Geometry: final body of the model. Coordinates: model frame, mm. Give positions to 0.01 mm unless a question says otherwise; leave off trailing zeros. Loops run counter-clockwise (first coordinate to the right, second up) from the corner with the lowest first, then second, coordinate; pieces in that order, holes last.
1. First-contact query: P1, Ø10, axis at y = 17, z = 9.5, coming from the -X side; P2, Ø8, axis at x = 371, z = 9, coming from the +Y side; P3, Ø4, axis at y = -11.5, z = 5.5, coming from the -X side. Flat tips, straight axial feed; report the tip coordinate or a pass-through.
2. Section A-A, the plane z = 19. Output: boundary loops of the cut face in (x, y).
3. Section B-B, the plane x = 319. Output: boundary loops of the cut face in (y, z), then the cut area to 3 significant figures.
4. Material intervals for line 1 along Y through (x, z) = (102.5, 24.5); line 2 along X through (y, z) = (-8, 21.25); line 3 along X through (y, z) = (1.5, 11.5), sorted ascending.
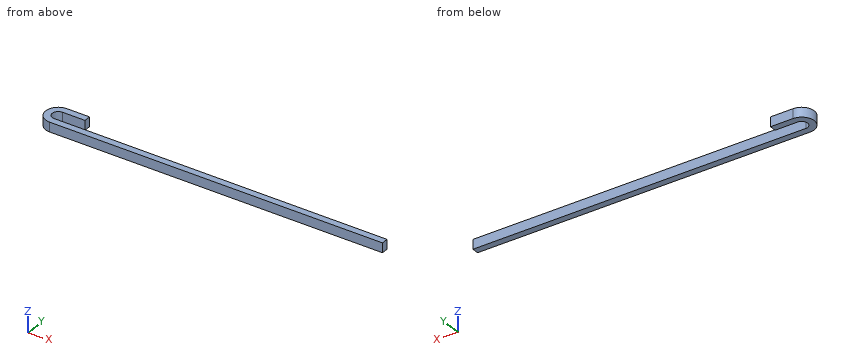
Autodesk Inventor part; units mm, degrees
ref_plane "YZ Plane" through (0, 0, 0) normal (1, 0, 0) x (0, 1, 0)
ref_plane "XZ Plane" through (0, 0, 0) normal (0, 1, 0) x (-1, 0, 0)
ref_plane "XY Plane" through (0, 0, 0) normal (0, 0, 1) x (1, 0, 0)
sketch "Sketch1" plane through (0, 0, 0) normal (0, 0, 1) x (1, 0, 0)
  circle A0 centre (0, 0) radius 38
  line L0 (0, -38) -> (1000, -38)
  line L1 (1000, -38) -> (1000, -18)
  line L2 (1000, -18) -> (0, -18)
  line L3 (0, -18) -> (0, -38)
  line L4 (0, 38) -> (68, 38)
  line L5 (68, 38) -> (68, 18)
  line L6 (68, 18) -> (0, 18)
  line L7 (0, 18) -> (0, 38)
  circle A1 centre (0, 0) radius 18
  dimension "d0" = 76
  dimension "d1" = 20
  dimension "d2" = 20
  dimension "d4" = 1000
  dimension "d7" = 68
extrude "Extrusion1" add sketch "Sketch1" along normal blind 29 contours L7 A1 L3 A0 | L4 L5 L6 A0 | A0 L6 L7 | L3 L2 A0 | A0 L2 L1 L0
properties part number "J15BF.1.20"
Answers below:
1. P1: stops at x = -36.06
1. P2: stops at y = -18
1. P3: stops at x = -36.79
2. outline: (0, -38) - (1000, -38) - (1000, -18) - (0, -18) arc R18 cw to (0, 18) - (68, 18) - (68, 38) - (0, 38) arc R38 ccw to start
3. outline: (-38, 0) - (-18, 0) - (-18, 29) - (-38, 29) - close
3. area: 580 mm2
4. line 1: y = -38 to -18
4. line 2: x = -37.15 to -16.12
4. line 3: x = -37.97 to -17.94
